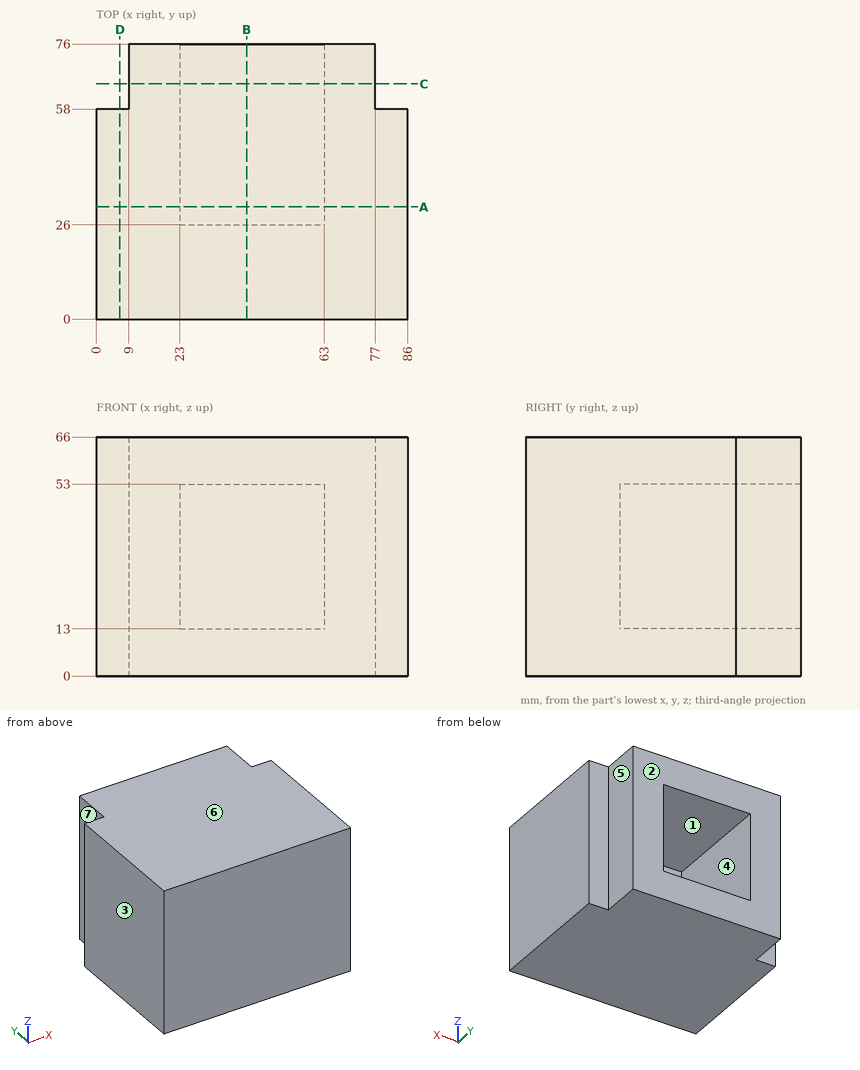
The figure shows three views and two pictorial views of one solid part (mm, origin at its lowest corner). Answer the questions. A direction names the side the tool comes from. Coordinates: 2 decimals unless noted, no trailing zeros. Loops run counter-clockwise (first coordinate to the right, second up) from the corner with the lowest first, then second, coordinate; pieces in that order, holes last. Notation, with made-up numbers: (-32.75, -38.5) -> (3.25, -38.5) arc R31 cw to (3.25, -11.5) -> close; hole circle Ø10 at (33, -29.5). An arc over 180 degrees is marked (long way). Use one line per item in the form item = value. Start each with the question number.
Item 1: The part is cut by section C-C on y = 65. Determine the outline of the cut face in (x, z).
Item 2: The part is cut by section B-B on x = 41.5. Determine the outline of the cut face in (y, z), then the cut area to 3 significant figures.
Item 3: Consider L1, parallel to X at y = 69.5, z = 20; L2, parallel to X at y = 54, z = 38.5; L3, parallel to Z at x = 43.5, y = 72.5. Determine where each line is inside the solid, lowest interval first. Write a range as [from, to].
Item 4: Flat-ended cylindrical pins translate along their axes: pin 1 Ø4.5 at (x, z) = (82, 25) entering from +Y; pin 2 Ø12 at (x, z) = (43, 34) entering from +Y. Find the tip coordinate at first contact, or state that the pin passes through.
Item 5: The part is cut by section A-A on y = 31. Determine the outline of the cut face in (x, z).
Item 6: A tool of negligible diameter and unlimited length cuts with its end or side. For the marked faces 5, 6 and 7, from which of +Z, -Z, +X, -X, +Y, -Y can it reach the whole face along a straight path? Write none if from no direction.
Item 7: The mould has two halves that part along X. Classify the marked faces 1, 2, 3 and 4: released by +X, released by -X, zero draft, split by the parting line, or undercut.
Item 8: The part is cut by section D-D on x = 6.5. Determine the outline of the cut face in (y, z), then the cut area to 3 significant figures.
Answer key:
q1.outline = (9, 0) -> (77, 0) -> (77, 66) -> (9, 66) -> close; hole (23, 13) -> (63, 13) -> (63, 53) -> (23, 53) -> close
q2.outline = (0, 0) -> (76, 0) -> (76, 13) -> (26, 13) -> (26, 53) -> (76, 53) -> (76, 66) -> (0, 66) -> close
q2.area = 3,020 mm2
q3.L1 = [9, 23], [63, 77]
q3.L2 = [0, 23], [63, 86]
q3.L3 = [0, 13], [53, 66]
q4.pin_1 = 58
q4.pin_2 = 26
q5.outline = (0, 0) -> (86, 0) -> (86, 66) -> (0, 66) -> close; hole (23, 13) -> (63, 13) -> (63, 53) -> (23, 53) -> close
q6.face_5 = +Z, -Z, +X, +Y
q6.face_6 = +Z, +X, -X, +Y, -Y
q6.face_7 = +Z, -Z, -X, +Y
q7.face_1 = undercut
q7.face_2 = zero draft
q7.face_3 = released by -X
q7.face_4 = undercut
q8.outline = (0, 0) -> (58, 0) -> (58, 66) -> (0, 66) -> close
q8.area = 3,830 mm2
